from build123d import *

# Parameters (mm, degrees)
SKETCH010_R      = 2.9
EXTRUDE010_DEPTH = 20
SKETCH009_W      = 19.993101
SKETCH009_H      = 12.095101
EXTRUDE009_DEPTH = 90


with BuildPart() as tornillos003:
    # Sketch010 (on Face4 of Extrude009) → Extrude010 (new body)
    with BuildSketch(Plane.XY.offset(20.871752)):
        with Locations((10, -80)):
            Circle(SKETCH010_R)
        with Locations((10, -45.010692)):
            Circle(SKETCH010_R)
        with Locations((10, -10.021384)):
            Circle(SKETCH010_R)
    extrude(amount=EXTRUDE010_DEPTH)


with BuildPart() as tornillos003_1:
    # Extrude010 placement: moved
    add(tornillos003.part.moved(Location((0, 0, -15))))


with BuildPart() as obj1:
    # Sketch009 → Extrude009 (new body)
    with BuildSketch(Plane.XZ):
        with Locations((9.99655, 14.824202)):
            Rectangle(SKETCH009_W, SKETCH009_H)
    extrude(amount=EXTRUDE009_DEPTH)

    # Cut003: cut Tornillos003
    add(tornillos003_1.part, mode=Mode.SUBTRACT)


with BuildPart() as obj1_1:
    # Cut003 placement: moved
    add(obj1.part.moved(Location((0, 90, 0))))


solid = obj1_1.part
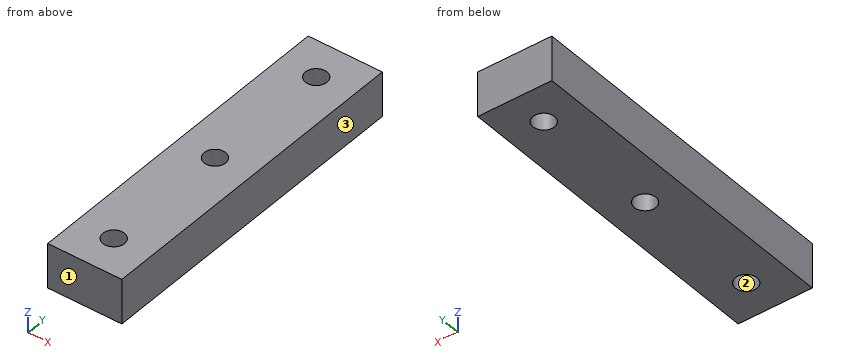
Verification items for the finished model (mm, model axes). Face numbers are marked on the shaded views. Coordinates: 2 decimals unless noted, no trailing zeros. Write each loop counter-clockwise with the first axis right and the second up, starting at its lowest first coordinate (ties: lowest second). Pieces come first, ordered by that corner, then holes. Notation, with made-up numbers: (-29.75, 71) - (-14.75, 71) arc R22 ccw to (-14.75, 81) - close; hole circle Ø10 at (10.5, 35). An arc over 180 degrees is marked (long way). Answer as a JSON object with one key per item and string values.
(1) Gauge pin test, flat ends, axial feed: pin 1 Ø3.5 at (x, y) = (10, 79.98) entering from -Z; pin 2 Ø4 at (x, z) = (9.5, 12.5) entering from -Y. Record the tip position at first contact, or that the pin passes through.
Report:
{"pin 1": "through", "pin 2": "y = 0"}
(2) Cross-section at B-B on x = 10. Record the cut outline in (y, z).
Report:
{"outline": "(0, 8.78) - (7.1, 8.78) - (7.1, 20.87) - (0, 20.87) - close; (12.9, 8.78) - (42.09, 8.78) - (42.09, 20.87) - (12.9, 20.87) - close; (47.89, 8.78) - (77.08, 8.78) - (77.08, 20.87) - (47.89, 20.87) - close; (82.88, 8.78) - (90, 8.78) - (90, 20.87) - (82.88, 20.87) - close"}
(3) Cross-section at D-D on y = 78. Record the cut outline in (x, z).
Report:
{"outline": "(0, 8.78) - (7.88, 8.78) - (7.88, 20.87) - (0, 20.87) - close; (12.12, 8.78) - (19.99, 8.78) - (19.99, 20.87) - (12.12, 20.87) - close"}
(4) Mould release check, pull along Y, two halves, no side actions. Record for the marked faces 1, 2 and 3: pulls with the +Y half, pulls with the -Y half, needs draft (parallel to the pull), parting line crosses it, or undercut.
Report:
{"face 1": "pulls with the -Y half", "face 2": "undercut", "face 3": "needs draft"}
(5) Thickness scan on line 1 along Y through (x, z) = (10, 15); line 2 along Y through (x, z) = (9, 15.5); line 3 along X through (y, z) = (80, 10.25). Record the ranges inside material, lowest first.
Report:
{"line 1": "0 to 7.1, 12.9 to 42.09, 47.89 to 77.08, 82.88 to 90", "line 2": "0 to 7.28, 12.72 to 42.27, 47.71 to 77.26, 82.7 to 90", "line 3": "0 to 7.1, 12.9 to 19.99"}
(6) Cross-section at C-C on z = 10.5. Record the cut outline in (x, y).
Report:
{"outline": "(0, 0) - (19.99, 0) - (19.99, 90) - (0, 90) - close; hole circle Ø5.8 at (10, 10); hole circle Ø5.8 at (10, 44.99); hole circle Ø5.8 at (10, 79.98)"}
(7) Cross-section at A-A on y = 10. Record the cut outline in (x, z).
Report:
{"outline": "(0, 8.78) - (7.1, 8.78) - (7.1, 20.87) - (0, 20.87) - close; (12.9, 8.78) - (19.99, 8.78) - (19.99, 20.87) - (12.9, 20.87) - close"}
